from build123d import *

# Parameters (mm, degrees)
SKIZZE1_R                       = 4
SKIZZE1_R_2                     = 1.5
AUFSATZ_LINEAR_AUSTRAGEN1_DEPTH = 4
FASE1_SIZE                      = 0.2
VERRUNDUNG1_R                   = 0.2


with BuildPart() as part:
    # Skizze1 → Aufsatz-Linear austragen1 (new body)
    with BuildSketch(Plane.XY):
        Circle(SKIZZE1_R)
        Circle(SKIZZE1_R_2, mode=Mode.SUBTRACT)
    extrude(amount=AUFSATZ_LINEAR_AUSTRAGEN1_DEPTH)

    # Fase1
    fase1_edges = [part.edges().sort_by_distance(p)[0] for p in [
        (-1.5, 0, 0),
        (-1.5, 0, 4),
    ]]
    chamfer(fase1_edges, length=FASE1_SIZE)

    # Verrundung1
    verrundung1_edges = [part.edges().sort_by_distance(p)[0] for p in [
        (-4, 0, 0),
        (-4, 0, 4),
    ]]
    fillet(verrundung1_edges, radius=VERRUNDUNG1_R)


solid = part.part
CAD build for the part. Positions are in the model's coordinates, mm. Give positions to 0.01 mm unless a question says otherwise; leave off trailing zeros. Loops run counter-clockwise (first coordinate to the right, second up) from the corner with the lowest first, then second, coordinate; pieces in that order, holes last. Notation, with made-up numbers: M 14,45 L 69,45 A26 cw 69,70 Z; hole C 21.25,26 d6. An arc over 180 degrees is marked long. Answer in a Markdown table with one row per item. Add a question column.
Item 1: Band-saw the part on A-A on y = 0. Give the cut face in (x, z), then the cut area to 3 significant figures.
Item 2: Drop flat-ended pins along their axis: P1, Ø1.5, axis at x = 1, z = 2.5, coming from the +Y side; P2, Ø1.5, axis at x = -3, z = 2.5, coming from the +Y side. Give the stop position or say it passes through.
Item 3: Mould opens along Y. For faces 1 (the face through (2, -1, 0)), 2 (the face through (-1.5, 0.07, 1.97)), 3 (the face through (-0.867, -3.905, 1.975)) say: +Y half, -Y half, draft (parallel to the pull), parting line (faces both ways), or undercut.
Item 4: Band-saw the part on C-C on z = 2.25. Give the cut face in (x, y), then the cut area to 3 significant figures.
Item 5: Probe probe 1 along Y at (x, z) = (0, 2.55); probe 2 along Y at (x, z) = (-0.5, 2.8); probe 3 along Y at (x, z) = (3.5, 0.25). List the from-to ranges inside material, lowest first.
Reply:
| question | item | result |
|---|---|---|
| 1 | outline | M -4,0.2 A0.2 ccw -3.8,0 L -1.7,0 L -1.5,0.2 L -1.5,3.8 L -1.7,4 L -3.8,4 A0.2 ccw -4,3.8 Z; M 1.5,0.2 L 1.7,0 L 3.8,0 A0.2 ccw 4,0.2 L 4,3.8 A0.2 ccw 3.8,4 L 1.7,4 L 1.5,3.8 Z |
| 1 | area | 19.9 mm^2 |
| 2 | P1 | stops at y = 3.99 |
| 2 | P2 | stops at y = 3.31 |
| 3 | face 1 | draft |
| 3 | face 2 | undercut |
| 3 | face 3 | parting line |
| 4 | outline | C 0,0 d8; hole C 0,0 d3 |
| 4 | area | 43.2 mm^2 |
| 5 | probe 1 | y = -4 to -1.5, 1.5 to 4 |
| 5 | probe 2 | y = -3.97 to -1.41, 1.41 to 3.97 |
| 5 | probe 3 | y = -1.94 to 1.94 |
